Autodesk Inventor part; units mm, degrees
ref_plane "YZ Plane" through (0, 0, 0) normal (1, 0, 0) x (0, 1, 0)
ref_plane "XZ Plane" through (0, 0, 0) normal (0, 1, 0) x (-1, 0, 0)
ref_plane "XY Plane" through (0, 0, 0) normal (0, 0, 1) x (1, 0, 0)
sketch "Sketch1" plane through (0, 0, 0) normal (0, 1, 0) x (-1, 0, 0)
  line L0 (15.25, -15.25) -> (-15.25, -15.25)
  line L1 (-15.25, 15.25) -> (15.25, 15.25)
  line L2 (15.25, -15.25) -> (-15.25, 15.25) construction
  line L3 (-15.25, -15.25) -> (15.25, 15.25) construction
  circle A0 centre (15.25, -15.25) radius 1.75
  circle A1 centre (-15.25, -15.25) radius 1.75
  circle A2 centre (15.25, 15.25) radius 1.75
  circle A3 centre (-15.25, 15.25) radius 1.75
  line L4 (21, -15.25) -> (-21, -15.25)
  line L5 (-21, -15.25) -> (-21, 15.25)
  line L6 (-21, 15.25) -> (21, 15.25)
  line L7 (21, 15.25) -> (21, -15.25)
  line L8 (21, -15.25) -> (-21, 15.25) construction
  line L9 (-21, -15.25) -> (21, 15.25) construction
  circle A4 centre (15.25, 15.25) radius 2.5
  circle A5 centre (-15.25, 15.25) radius 2.5
  circle A6 centre (-15.25, -15.25) radius 2.5
  circle A7 centre (15.25, -15.25) radius 2.5
  line L10 (22.5, -17.75) -> (-22.5, -17.75)
  line L11 (-22.5, -17.75) -> (-22.5, 17.75)
  line L12 (-22.5, 17.75) -> (22.5, 17.75)
  line L13 (22.5, 17.75) -> (22.5, -17.75)
  line L14 (22.5, -17.75) -> (-22.5, 17.75) construction
  line L15 (-22.5, -17.75) -> (22.5, 17.75) construction
  point P0 (0, 0)
  point P1 (12.75, 15.25)
  point P2 (17.75, 15.25)
  point P3 (17.75, -15.25)
  point P4 (12.75, -15.25)
  point P5 (-12.75, -15.25)
  point P6 (-17.75, -15.25)
  point P7 (-17.75, 15.25)
  point P8 (-12.75, 15.25)
  dimension "d0" = 30.5
  dimension "d1" = 30.5
  dimension "d2" = 3.5
  dimension "d3" = 3.5
  dimension "d4" = 3.5
  dimension "d5" = 3.5
  dimension "d6" = 42
  dimension "d7" = 5
  dimension "d8" = 5
  dimension "d9" = 5
  dimension "d10" = 5
  dimension "d11" = 45
sketch "Sketch2" plane through (0, 0, 0) normal (0, 1, 0) x (-1, 0, 0)
  line L0 (30, -10) -> (-30, -10)
  line L1 (-30, -10) -> (-30, 10)
  line L2 (-30, 10) -> (30, 10)
  line L3 (30, 10) -> (30, -10)
  line L4 (30, -10) -> (-30, 10) construction
  line L5 (-30, -10) -> (30, 10) construction
  line L6 (2.5, -2.5) -> (-2.5, -2.5)
  line L7 (-2.5, -2.5) -> (-2.5, 2.5)
  line L8 (-2.5, 2.5) -> (2.5, 2.5)
  line L9 (2.5, 2.5) -> (2.5, -2.5)
  line L10 (2.5, -2.5) -> (-2.5, 2.5) construction
  line L11 (-2.5, -2.5) -> (2.5, 2.5) construction
  line L12 (0, 0) -> (53.033, 53.033)
  line L13 (0, 0) -> (53.033, -53.033)
  line L14 (0, 0) -> (-53.033, -53.033)
  line L15 (0, 0) -> (-53.033, 53.033)
  circle A0 centre (-53.033, -53.033) radius 32.5
  circle A1 centre (53.033, -53.033) radius 32.5
  circle A2 centre (53.033, 53.033) radius 32.5
  circle A3 centre (-53.033, 53.033) radius 32.5
  circle A4 centre (-53.033, 53.033) radius 7.5
  circle A5 centre (53.033, 53.033) radius 7.5
  circle A6 centre (-53.033, -53.033) radius 7.5
  circle A7 centre (53.033, -53.033) radius 7.5
  line L16 (34.5, 21) -> (-34.5, 21)
  line L17 (-34.5, 21) -> (-34.5, -21)
  line L18 (-34.5, -21) -> (34.5, -21)
  line L19 (34.5, -21) -> (34.5, 21)
  line L20 (34.5, 21) -> (-34.5, -21) construction
  line L21 (-34.5, 21) -> (34.5, -21) construction
  line L22 (34.5, -21) -> (58.6289, -48.0394)
  line L23 (58.6289, -48.0394) -> (47.4371, -58.0266)
  line L24 (47.4371, -58.0266) -> (10.4105, -21)
  line L25 (-34.5, -21) -> (-58.6289, -48.0394)
  line L26 (-47.4371, -58.0266) -> (-10.4105, -21)
  line L27 (-34.5, 21) -> (-58.6289, 48.0394)
  line L28 (-47.4371, 58.0266) -> (-10.4105, 21)
  line L29 (47.4371, 58.0266) -> (10.4105, 21)
  line L30 (34.5, 21) -> (58.6289, 48.0394)
  line L31 (15.25, 15.25) -> (-15.25, 15.25)
  line L32 (-15.25, 15.25) -> (-15.25, -15.25)
  line L33 (-15.25, -15.25) -> (15.25, -15.25)
  line L34 (15.25, -15.25) -> (15.25, 15.25)
  line L35 (15.25, 15.25) -> (-15.25, -15.25) construction
  line L36 (-15.25, 15.25) -> (15.25, -15.25) construction
  circle A8 centre (15.25, -15.25) radius 1.75
  circle A9 centre (-15.25, -15.25) radius 1.75
  circle A10 centre (15.25, 15.25) radius 1.75
  circle A11 centre (-15.25, 15.25) radius 1.75
  circle A12 centre (53.033, 53.033) radius 4.5
  circle A13 centre (-53.033, 53.033) radius 4.5
  circle A14 centre (-53.033, -53.033) radius 4.5
  circle A15 centre (53.033, -53.033) radius 4.5
  line L37 (57.533, 53.033) -> (48.533, 53.033)
  line L38 (53.033, 57.533) -> (53.033, 48.533)
  circle A16 centre (57.533, 53.033) radius 1.25
  circle A17 centre (53.033, 48.533) radius 1.25
  circle A18 centre (48.533, 53.033) radius 1.25
  circle A19 centre (53.033, 57.533) radius 1.25
  circle A20 centre (-53.033, 57.533) radius 1.25
  circle A21 centre (-53.033, 48.533) radius 1.25
  circle A22 centre (-57.533, 53.033) radius 1.25
  circle A23 centre (-48.533, 53.033) radius 1.25
  circle A24 centre (-57.533, -53.033) radius 1.25
  circle A25 centre (-48.533, -53.033) radius 1.25
  circle A26 centre (-53.033, -57.533) radius 1.25
  circle A27 centre (-53.033, -48.533) radius 1.25
  circle A28 centre (48.533, -53.033) radius 1.25
  circle A29 centre (57.533, -53.033) radius 1.25
  circle A30 centre (53.033, -57.533) radius 1.25
  circle A31 centre (53.033, -48.533) radius 1.25
  circle A32 centre (53.033, 53.033) radius 2
  circle A33 centre (-53.033, 53.033) radius 2
  circle A34 centre (-53.033, -53.033) radius 2
  circle A35 centre (53.033, -53.033) radius 2
  dimension "d14" = 60
  dimension "d15" = 20
  dimension "d16" = 5
  dimension "d17" = 5
  dimension "d20" = 75
  dimension "d21" = 75
  dimension "d22" = 75
  dimension "d23" = 65
  dimension "d24" = 65
  dimension "d25" = 65
  dimension "d26" = 65
  dimension "d27" = 75
  dimension "d28" = 15
  dimension "d29" = 15
  dimension "d31" = 15
  dimension "d32" = 15
  dimension "d33" = 69
  dimension "d34" = 42
  dimension "d35" = 30.5
  dimension "d36" = 30.5
  dimension "d37" = 3.5
  dimension "d38" = 3.5
  dimension "d39" = 3.5
  dimension "d40" = 3.5
  dimension "d41" = 9
  dimension "d42" = 9
  dimension "d43" = 9
  dimension "d44" = 9
  dimension "d45" = 2.5
  dimension "d46" = 2.5
  dimension "d47" = 2.5
  dimension "d48" = 2.5
  dimension "d49" = 2.5
  dimension "d50" = 2.5
  dimension "d51" = 2.5
  dimension "d52" = 2.5
  dimension "d53" = 2.5
  dimension "d54" = 2.5
  dimension "d55" = 2.5
  dimension "d56" = 2.5
  dimension "d57" = 2.5
  dimension "d58" = 2.5
  dimension "d59" = 2.5
  dimension "d60" = 2.5
  dimension "d61" = 4
  dimension "d62" = 4
  dimension "d63" = 4
  dimension "d64" = 4
extrude "Extrusion2" add sketch "Sketch2" along normal blind 3.5 contours L3 L2 L34 A10 L12 L16 L19 L18 L13 A8 L0 | L34 A8 L13 L0 | L13 A8 L33 A9 L14 L0 | L2 L12 A10 L34 | L14 A9 L32 L0 | L2 L15 A11 L31 A10 L12 | L32 A9 L14 L18 L17 L16 L15 A11 L2 L1 L0 | A8 L13 L18 L14 A9 L33 | L2 L32 A11 L15 | L18 L22 A1 L13 | L13 A1 L24 L18 | L31 A11 L15 L16 L12 A10 | A1 L22 A7 L13 | L13 A7 L24 A1 | L16 L29 A2 L12 | L12 A2 L30 L16 | L18 L26 A0 L14 | L14 A0 L25 L18 | A7 L23 A15 A31 L13 | L13 A15 A28 L23 A7 | A2 L29 A5 L12 | L12 A5 L30 A2 | L16 L27 A3 L15 | L15 A3 L28 L16 | A0 L26 A6 L14 | L14 A6 L25 A0 | A15 A31 L23 A35 L13 | L13 A35 L23 A15 A28 | A7 L23 A15 A30 A29 | A12 A18 L37 A32 L12 | L12 A32 L38 A17 A12 | A5 | A3 L27 A4 L15 | L15 A4 L28 A3 | A14 A25 A26 A24 A27 | A6 | A15 A29 A30 L23 A35 | A13 A21 A22 A20 A23 | A4 | L37 A18 A12 A19 L38 A32 | A32 L37 A16 A12 A17 L38 | A32 L38 A19 A12 A16 L37
fillet "Fillet1" radius 8 8 edges at (-10.4105, 1.75, 21) (-34.5, 1.75, 21) (-34.5, 1.75, -21) (34.5, 1.75, -21) (10.4105, 1.75, -21) (10.4105, 1.75, 21) (34.5, 1.75, 21) (-10.4105, 1.75, -21)
fillet "Fillet2" radius 2 4 edges at (-30, 1.75, -10) (30, 1.75, -10) (30, 1.75, 10) (-30, 1.75, 10)
properties part number "Crazyflie Bolt Mount"
Build history of the part. All positions in model axes, mm. A direction names the side the tool comes from. Give positions to 0.01 mm unless a question says otherwise; leave off trailing zeros. Loops run counter-clockwise (first coordinate to the right, second up) from the corner with the lowest first, then second, coordinate; pieces in that order, holes last. Notation, with made-up numbers: (-8.5, 0) - (15.5, 0) arc R21 ccw to (15.5, 37) - close; hole circle Ø1 at (48, 64.5). An arc over 180 degrees is marked (long way). Write item = value, one per line. Start each with the question number.
1) Pull direction X, two halves, no side cores. Call faces 1 (the flat face through (5, 0, -13)), 2 (the flat face through (-47.425, 1.726, -35.484)), 3 (the flat face through (47.425, 1.726, -35.484)), 4 (the flat face through (0, 2, 21)): +X half, -X half, draft (parallel to the pull), parting line (faces both ways), or undercut.
2) Band-saw the part on D-D on z = 3. Give the cut face in (x, y).
3) Band-saw the part on B-B on z = -15.25. Give the cut face in (x, y), plus the area to 3 significant figures.
4) Band-saw the part on A-A on x = 1.5. Give the cut face in (y, z).
5) Tool access for faces 5 (the flat face through (-30, 2, 0)), 6 (the flat face through (-30.34, 1.73, 40.93)), 7 (the cylindrical face through (35.04, 1.77, -20.84)), 8 (the flat face through (-47.425, 1.726, 35.484)): list every direction of +Z, -Z, +X, -X, +Y, -Y with a clear straight run to the whole face (end or side of a thin tool).
6) Band-saw the part on C-C on x = -15.25. Give the cut face in (y, z), plus the area to 3 significant figures.
7) Drop flat-ended pins along their axis: pin 1 Ø2 at (x, y) = (-11.5, 2.5) entering from -Z; pin 2 Ø1 at (y, z) = (2.5, -4) entering from +X. Give the stop position or say it passes through.
8) Probe probe 1 along Z at (x, y) = (-48.5, 0.9); probe 2 along X at (y, z) = (1.55, -14.5); probe 3 along Z at (x, y) = (2, 2.85). List the from-to ranges inside material, lowest first. Write a range as from..to.
Final values:
q1.face_1 = draft
q1.face_2 = -X half
q1.face_3 = +X half
q1.face_4 = undercut
q2.outline = (-34.5, 0) - (-30, 0) - (-30, 3.5) - (-34.5, 3.5) - close; (30, 0) - (34.5, 0) - (34.5, 3.5) - (30, 3.5) - close
q3.outline = (-34.5, 0) - (-17, 0) - (-17, 3.5) - (-34.5, 3.5) - close; (-13.5, 0) - (13.5, 0) - (13.5, 3.5) - (-13.5, 3.5) - close; (17, 0) - (34.5, 0) - (34.5, 3.5) - (17, 3.5) - close
q3.area = 217 mm²
q4.outline = (0, -21) - (3.5, -21) - (3.5, -10) - (0, -10) - close; (0, 10) - (3.5, 10) - (3.5, 21) - (0, 21) - close
q5.face_5 = +Y, -Y
q5.face_6 = +Z, +Y, -Y
q5.face_7 = +X, +Y, -Y
q5.face_8 = -X, +Y, -Y
q6.outline = (0, -25.84) - (3.5, -25.84) - (3.5, -17) - (0, -17) - close; (0, -13.5) - (3.5, -13.5) - (3.5, -10) - (0, -10) - close; (0, 10) - (3.5, 10) - (3.5, 13.5) - (0, 13.5) - close; (0, 17) - (3.5, 17) - (3.5, 25.84) - (0, 25.84) - close
q6.area = 86.4 mm²
q7.pin_1 = -23.1
q7.pin_2 = 34.5
q8.probe_1 = -59.01..-54.28, -51.78..-36.69, 36.69..51.78, 54.28..59.01
q8.probe_2 = -34.5..-16.83, -13.67..13.67, 16.83..34.5
q8.probe_3 = -21..-10, 10..21
